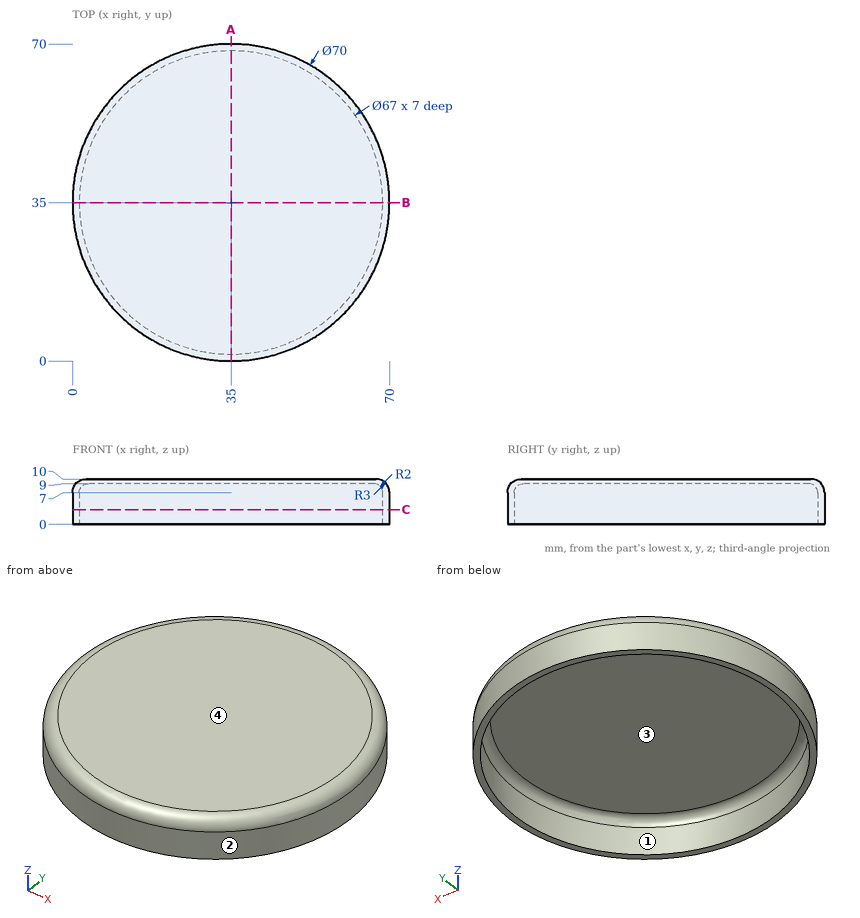
Source: three-view drawing plus pictorial views. Frame: mm from the lowest corner of the part. Round coordinates to 2 decimals unless told otherwise and drop trailing zeros. Order: outer loops, then holes, each group sorted by start corner. A loop starts at its lowest first (then second) coordinate and runs counter-clockwise, first axis right, second up. Notation, with made-up numbers: (10, -26.5) -> (63, -26.5) arc R23 ccw to (63, -9.5) -> close; hole circle Ø10 at (61.25, 85). An arc over 180 degrees is marked (long way). Use CSV: the item, a comma, the result in double quotes. Start each with the question number.
1) First-contact query: pin 1 Ø3 at (y, z) = (12, 6) entering from +X; pin 2 Ø4 at (y, z) = (19, 4) entering from +X; pin 3 Ø1.5 at (y, z) = (13.5, 7.5) entering from +X. Flat tips, straight axial feed; report the tip coordinate or a pass-through.
2) Section A-A (x = 35). Return the cut outline in (y, z).
3) Section C-C (z = 3.25). Return the cut outline in (x, y), and give its area (3 significant figures).
4) Draft query along X for the marked faces 1, 2, 3 and 4. Return one class per face: +X half, -X half, draft (parallel to the pull), parting line (faces both ways), or undercut.
5) Material intervals for line 1 along Y through (x, z) = (35, 2.25); line 2 along Z through (x, y) = (64.5, 44.5); line 3 along X through (y, z) = (53, 8.25), sorted ascending. Write a range as from..to.
Returned:
1,pin 1,"stops at x = 62.62"
1,pin 2,"stops at x = 67.08"
1,pin 3,"stops at x = 63.15"
2,outline,"(0, 0) -> (1.5, 0) -> (1.5, 7) arc R2 cw to (3.5, 9) -> (66.5, 9) arc R2 cw to (68.5, 7) -> (68.5, 0) -> (70, 0) -> (70, 7) arc R3 ccw to (67, 10) -> (3, 10) arc R3 ccw to (0, 7) -> close"
3,outline,"circle Ø70 at (35, 35); hole circle Ø67 at (35, 35)"
3,area,"323 mm²"
4,face 1,"undercut"
4,face 2,"parting line"
4,face 3,"undercut"
4,face 4,"draft"
5,line 1,"y = 0..1.5, 68.5..70"
5,line 2,"z = 9..10"
5,line 3,"x = 5.3..7.27, 62.73..64.7"
